```python
from build123d import *

# Parameters (mm, degrees)
SKETCH2_W                   = 508
SKETCH2_H                   = 127
BOSS_EXTRUDE1_DEPTH         = 63.5
SKETCH3_W                   = 127
SKETCH3_H                   = 127
BOSS_EXTRUDE2_DEPTH         = 444.5
SKETCH4_W                   = 31.75
SKETCH4_H                   = 31.75
CUT_EXTRUDE1_DEPTH          = 38.1
SKETCH5_R                   = 12.7
CUT_EXTRUDE2_DEPTH          = 50.8
SKETCH6_W                   = 63.5
SKETCH6_H                   = 63.5
CUT_EXTRUDE3_DEPTH          = 63.5
F_1_4_0_25_DIAMETER_HOLE1_D = 6.35
BOSS_EXTRUDE3_DEPTH         = 6.35
EXTRUDE_THIN1_START         = -6.35
EXTRUDE_THIN1_DEPTH         = 6.35
SKETCH12_R                  = 3.175
CUT_EXTRUDE4_DEPTH          = 603.413894262


# Read off the part's stored shape, not the designer's step: Extrude-Thin1
with BuildPart() as part:
    # Sketch2 → Boss-Extrude1 (new body)
    with BuildSketch(Plane(origin=(0, 0, 0), x_dir=(0, 0, -1), z_dir=(1, 0, 0))):
        Rectangle(SKETCH2_W, SKETCH2_H)
    extrude(amount=BOSS_EXTRUDE1_DEPTH)

    # Sketch3 → Boss-Extrude2 (add)
    with BuildSketch(Plane(origin=(63.5, 0, 0), x_dir=(0, 0, -1), z_dir=(1, 0, 0))):
        Rectangle(SKETCH3_W, SKETCH3_H)
    extrude(amount=BOSS_EXTRUDE2_DEPTH)

    # Sketch4 → Cut-Extrude1 (cut)
    with BuildSketch(Plane.ZY):
        Rectangle(SKETCH4_W, SKETCH4_H)
    extrude(amount=-CUT_EXTRUDE1_DEPTH, mode=Mode.SUBTRACT)

    # Sketch5 → Cut-Extrude2 (cut)
    with BuildSketch(Plane.ZY.offset(-38.1)):
        Circle(SKETCH5_R)
    extrude(amount=-CUT_EXTRUDE2_DEPTH, mode=Mode.SUBTRACT)

    # Sketch6 → Cut-Extrude3 (cut)
    with BuildSketch(Plane(origin=(0, 63.5, 0), x_dir=(1, 0, 0), z_dir=(0, 1, 0))):
        with Locations((377.19, 0)):
            Rectangle(SKETCH6_W, SKETCH6_H)
    extrude(amount=-CUT_EXTRUDE3_DEPTH, mode=Mode.SUBTRACT)

    # 1/4 (0.25) Diameter Hole1 (through all)
    with Locations(Plane.XY.offset(63.5)):
        with Locations((476.25, -31.75), (412.75, -31.75), (412.75, 31.75), (476.25, 31.75)):
            Hole(F_1_4_0_25_DIAMETER_HOLE1_D / 2)

    # Sketch10 → Boss-Extrude3 (add)
    with BuildSketch(Plane.XZ.offset(63.5)):
        Polygon((63.5, 254), (406.4, 63.5), (368.3, 63.5), (63.5, 232.833333333), align=None)
    boss_extrude3 = extrude(amount=-BOSS_EXTRUDE3_DEPTH)

    # Mirror1: Boss-Extrude3 across plane
    add(boss_extrude3.mirror(Plane.XY))

    # Extrude-Thin1 outline → Extrude-Thin1 (add)
    with BuildSketch(Plane(origin=(0, -57.15, 0), x_dir=(1, 0, 0), z_dir=(0, 1, 0)).offset(EXTRUDE_THIN1_START)):
        Polygon((81.701018612, -63.5), (76.2, -63.5), (227.001797407, -141.999001441), (229.66281775, -140.520656806), align=None)
        Polygon((215.9, -148.166666667), (63.5, -63.5), (63.5, -66.405655618), (213.284909944, -149.619494475), align=None)
        Polygon((204.798202593, -154.334331893), (63.5, -76.2), (63.5, -79.10247771), (202.17989093, -155.788949483), align=None)
    extrude_thin1 = extrude(amount=EXTRUDE_THIN1_DEPTH)

    # Mirror2: Extrude-Thin1 across plane
    add(extrude_thin1.mirror(Plane.XY))

    # Sketch12 → Cut-Extrude4 (cut, through all)
    with BuildSketch(Plane.XY.offset(63.5)):
        with Locations((177.8, 20.701)):
            Circle(SKETCH12_R)
        with Locations((177.8, -20.701)):
            Circle(SKETCH12_R)
        with Locations((330.2, 20.701)):
            Circle(SKETCH12_R)
        with Locations((330.2, -20.701)):
            Circle(SKETCH12_R)
    extrude(amount=-CUT_EXTRUDE4_DEPTH, mode=Mode.SUBTRACT)


solid = part.part
```
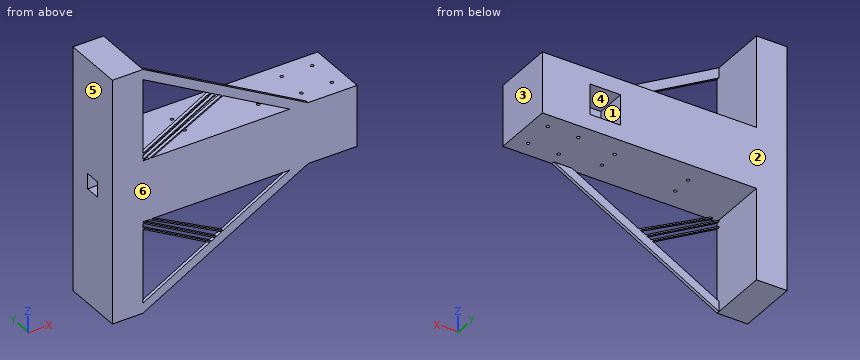
The model under review builds one solid part; all positions refer to its coordinate system, in mm. Face numbers are marked on the shaded views. A direction names the side the tool comes from. Coordinates: 2 decimals unless noted, no trailing zeros. Order: outer loops, then holes, each group sorted by start corner. A loop starts at its lowest first (then second) coordinate and runs counter-clockwise, first axis right, second up. Notation, with made-up numbers: M -33.5,72.25 L -24.5,72.25 A17 cw -24.5,80.25 Z; hole C 12,-23 d1. An arc over 180 degrees is marked long. One line per question, with ' | ' between items.
(1) Insertion check: pin 1 (7.5 mm diameter, centred on x = 412.75, y = 31.75, fed in from +Z); pin 2 (4 mm diameter, centred on x = 330.2, y = -20.701, fed in from -Z); pin 3 (1.5 mm diameter, centred on y = -28.5, z = -126.5, fed in from +X); pin 4 (8 mm diameter, centred on x = 412.5, y = 48.5, fed in from -Z). Each pin has a flat end and moves straight along its axis. Give the tip position at first contact, or say it passes through.
Geometry results:
pin 1: stops at z = 63.5 | pin 2: passes through | pin 3: stops at x = 63.5 | pin 4: stops at z = -63.5
(2) For probe 1 along X at (y, z) = (-31, 37); probe 2 along Y at (x, z) = (177.8, -12); probe 3 along Y at (x, z) = (412.75, -12) (3 decimals), list the stretches that pass through material, from the lowest coordinate up. Write a range as from..to.
Geometry results:
probe 1: x = 0..409.66, 415.84..473.16, 479.34..508 | probe 2: y = -63.5..-23.88, -17.53..17.53, 23.88..63.5 | probe 3: y = -63.5..-34.925, -28.575..28.575, 34.925..63.5
(3) The part is to be moulded in two halves that separate along X. For the marked faces 3, 4, 5 and 6, say which applies: +X half, -X half, draft (parallel to the pull), parting line (faces both ways), or undercut.
Geometry results:
face 3: +X half | face 4: undercut | face 5: -X half | face 6: draft
(4) Add section C-C, the plane y = -51. Write out the cut boundary in (x, z).
Geometry results:
outline: M 0,-254 L 63.5,-254 L 63.5,-63.5 L 508,-63.5 L 508,63.5 L 63.5,63.5 L 63.5,254 L 0,254 Z
(5) Machinability: for the marked faces 1 and 2, which of the approach directions +Z, -Z, +X, -X, +Y, -Y give a long, thin tool a straight path to every point of the face, cutting with its end or side? Answer none if there is none.
Geometry results:
face 1: +Y | face 2: +Z, -Z, +X, -X, +Y
(6) Add section B-B, the plane y = 45.5. Write out the cut boundary in (x, z).
Geometry results:
outline: M 0,-254 L 63.5,-254 L 63.5,-63.5 L 508,-63.5 L 508,63.5 L 63.5,63.5 L 63.5,254 L 0,254 Z; hole M 345.44,-31.75 L 408.94,-31.75 L 408.94,31.75 L 345.44,31.75 Z
(7) Add section D-D, the plane z = -4. State how many separate pieces and enclosed holes the cut face has, then the cut area to 3 significant figures.
Geometry results:
separate pieces: 1 | enclosed holes: 8 | area: 57,800 mm²
(8) Add section A-A, the plane z = -179. Write out the cut boundary in (x, y), then the cut area to 3 significant figures.
Geometry results:
outline: M 0,-63.5 L 63.5,-63.5 L 63.5,63.5 L 0,63.5 Z; M 160.4,-63.5 L 198.5,-63.5 L 198.5,-57.15 L 160.4,-57.15 Z | area: 8,310 mm²
